from build123d import *

# Parameters (mm, degrees)
CROQUIS1_R              = 2
CROQUIS1_W              = 3
CROQUIS1_H              = 10
SALIENTE_EXTRUIR1_DEPTH = 3


with BuildPart() as part:
    # Croquis1 → Saliente-Extruir1 (new body)
    with BuildSketch(Plane(origin=(0, 0, 0), x_dir=(1, 0, 0), z_dir=(0, 1, 0))):
        with BuildLine():
            Line((-29.945152174, -20.924198867), (-29.945152174, 62.5))
            Line((-29.945152174, 62.5), (-4.069135421, 62.5))
            Line((-4.069135421, 62.5), (-4.069135421, 59.5))
            Line((-4.069135421, 59.5), (5.930864579, 59.5))
            Line((5.930864579, 59.5), (5.930864579, 62.5))
            Line((5.930864579, 62.5), (30.054847826, 62.5))
            Line((30.054847826, 62.5), (30.054847826, -20.924198867))
            ThreePointArc((30.054847826, -20.924198867), (0.054847826, -94.111194706), (-29.945152174, -20.924198867))
        make_face()
        with Locations(Location((-24.3, 37.439181633, 0), (0, 0, 270))):
            Circle(CROQUIS1_R, mode=Mode.SUBTRACT)
        with Locations((28.554847826, -55)):
            Rectangle(CROQUIS1_W, CROQUIS1_H, mode=Mode.SUBTRACT)
        with Locations((-28.445152174, -55)):
            Rectangle(CROQUIS1_W, CROQUIS1_H, mode=Mode.SUBTRACT)
        with BuildLine():
            Line((8.554847826, -75.182623358), (-8.445152174, -75.182623358))
            ThreePointArc((-8.445152174, -75.182623358), (-9.945152174, -76.682623358), (-8.445152174, -78.182623358))
            Line((-8.445152174, -78.182623358), (8.554847826, -78.182623358))
            ThreePointArc((8.554847826, -78.182623358), (10.054847826, -76.682623358), (8.554847826, -75.182623358))
        make_face(mode=Mode.SUBTRACT)
        with BuildLine():
            Line((8.554847826, -81.682623358), (-8.445152174, -81.682623358))
            ThreePointArc((-8.445152174, -81.682623358), (-9.945152174, -83.182623358), (-8.445152174, -84.682623358))
            Line((-8.445152174, -84.682623358), (8.554847826, -84.682623358))
            ThreePointArc((8.554847826, -84.682623358), (10.054847826, -83.182623358), (8.554847826, -81.682623358))
        make_face(mode=Mode.SUBTRACT)
        with BuildLine():
            ThreePointArc((25.157138558, -76.471354215), (32.85257123, -64.954325332), (35.554847826, -51.369063483))
            ThreePointArc((35.554847826, -51.369063483), (37.054847826, -49.869063483), (38.554847826, -51.369063483))
            ThreePointArc((38.554847826, -51.369063483), (35.624209827, -66.102375629), (27.278458901, -78.592674559))
            ThreePointArc((27.278458901, -78.592674559), (25.157138558, -78.592674559), (25.157138558, -76.471354215))
        make_face(mode=Mode.SUBTRACT)
        with BuildLine():
            ThreePointArc((-35.445152174, -51.369063483), (-32.742875579, -64.954325332), (-25.047442907, -76.471354215))
            ThreePointArc((-25.047442907, -76.471354215), (-25.047442907, -78.592674559), (-27.16876325, -78.592674559))
            ThreePointArc((-27.16876325, -78.592674559), (-35.514514176, -66.102375629), (-38.445152174, -51.369063483))
            ThreePointArc((-38.445152174, -51.369063483), (-36.945152174, -49.869063483), (-35.445152174, -51.369063483))
        make_face(mode=Mode.SUBTRACT)
    extrude(amount=SALIENTE_EXTRUIR1_DEPTH)


solid = part.part
For this review, take the finished solid that the model builds, in its own axes (mm). A direction names the side the tool comes from. Give positions to 0.01 mm unless a question says otherwise; leave off trailing zeros. Loops run counter-clockwise (first coordinate to the right, second up) from the corner with the lowest first, then second, coordinate; pieces in that order, holes last.
Item 1: Tool access review of faces 4 (the flat face through (-28, 1, 60)), 5 (the flat face through (-29.945, 1, -20)), 6 (the flat face through (1, 1, -59.5)), 7 (the flat face through (30.055, 1, -21)), 8 (the flat face through (-17, 1, -62.5)): name each direction out of +Z, -Z, +X, -X, +Y, -Y from which nothing blocks a thin tool from reaching the whole face with its end or side.
Item 2: Insertion check: pin 1 (0.9 mm diameter, centred on y = 1.5, z = -61.5, fed in from -X); pin 2 (1 mm diameter, centred on y = 1.5, z = -6.5, fed in from +X); pin 3 (0.9 mm diameter, centred on x = -2, y = 1, fed in from -Z). Each pin has a flat end and moves straight along its axis. Give the tip position at first contact, or say it passes through.
Item 3: Draft analysis for pull direction Z (two halves, no side actions). For faces 1 (the flat face through (30.055, 1, 55)), 2 (the flat face through (18, 1, -62.5)), 3 (the flat face through (-4.069, 1, -61)), state which applies: +Z half, -Z half, draft (parallel to the pull), parting line (faces both ways), or undercut.
Item 4: Take a section at A-A, the plane x = 0.5. State the section outline as (y, z) points, and give its area (3 significant figures).
Item 5: Take a section at C-C, the plane y = 1.75. Give the number of separate pieces and of enclosed holes in the cut face, and give its area (3 significant figures).
Item 6: Take a section at D-D, the plane z = 18. State the section outline as (x, y) points, and give its area (3 significant figures).
Item 7: For line 1 along Z through (x, y) = (1, 2.15); line 2 along X through (y, z) = (1.2, 78); line 3 along X through (y, z) = (1.45, 75.5), list the stretches that pass through material, from the lowest coordinate up.
Item 8: Take a section at B-B, the plane z = 73.5. State the section outline as (x, y) points, and give its area (3 significant figures).
Calculated:
1. face 4: +Y, -Y
1. face 5: -Z, -X, +Y, -Y
1. face 6: -Z, +Y, -Y
1. face 7: -Z, +X, +Y, -Y
1. face 8: -Z, +X, -X, +Y, -Y
2. pin 1: stops at x = -29.95
2. pin 2: stops at x = 30.05
2. pin 3: stops at z = -59.5
3. face 1: undercut
3. face 2: -Z half
3. face 3: draft
4. outline: (0, -59.5) - (3, -59.5) - (3, 75.18) - (0, 75.18) - close; (0, 78.18) - (3, 78.18) - (3, 81.68) - (0, 81.68) - close; (0, 84.68) - (3, 84.68) - (3, 94.11) - (0, 94.11) - close
4. area: 443 mm2
5. separate pieces: 1
5. enclosed holes: 7
5. area: 9,830 mm2
6. outline: (-29.95, 0) - (30.05, 0) - (30.05, 3) - (-29.95, 3) - close
6. area: 180 mm2
7. line 1: z = -59.5 to 75.18, 78.18 to 81.68, 84.68 to 94.1
7. line 2: x = -33.38 to -27.75, -24.68 to -9.16, 9.27 to 24.79, 27.86 to 33.49
7. line 3: x = -35.22 to -29.94, -25.98 to -9.37, 9.48 to 26.09, 30.05 to 35.33
8. outline: (-36.51, 0) - (-31.45, 0) - (-31.45, 3) - (-36.51, 3) - close; (-27.7, 0) - (27.81, 0) - (27.81, 3) - (-27.7, 3) - close; (31.56, 0) - (36.62, 0) - (36.62, 3) - (31.56, 3) - close
8. area: 197 mm2
